Read the model definition and answer for the solid it produces. Units are mm, in the model's axes. Face numbers are marked on the shaded views. A direction names the side the tool comes from. Coordinates: 2 decimals unless noted, no trailing zeros. Write each loop counter-clockwise with the first axis right and the second up, starting at its lowest first coordinate (ties: lowest second). Pieces come first, ordered by that corner, then holes. Notation, with made-up numbers: (82.25, 72.5) -> (108.25, 72.5) arc R25 cw to (108.25, 96.5) -> close; hole circle Ø10 at (5, -0.75). An arc over 180 degrees is marked (long way). Use CSV: the item, a comma, the result in double quotes.
from build123d import *

# Parameters (mm, degrees)
F0_W     = 15
F0_H     = 18
F0_R     = 6
F0_W_2   = 10.2
F0_H_2   = 3.3
F1_DEPTH = 50
F2_D     = 12
F2_DEPTH = 45
F2_TIP   = 3.6051637142
F3_R     = 5
F4_R     = 5
F6_W     = 10.2
F6_H     = 3.3
F7_DEPTH = 40


with BuildPart() as f1:
    # F0 (on Top) → F1 (new body)
    with BuildSketch(Plane.XY):
        with Locations((0, 1.5)):
            Rectangle(F0_W, F0_H)
        Circle(F0_R, mode=Mode.SUBTRACT)
        with Locations((-0.15, 8.3)):
            Rectangle(F0_W_2, F0_H_2, mode=Mode.SUBTRACT)
        with Locations((-0.15, 8.3)):
            Rectangle(F0_W_2, F0_H_2)
        Circle(F0_R)
    extrude(amount=F1_DEPTH)

    # F2
    with Locations(Plane(origin=(0, 0, 0), x_dir=(1, 0, 0), z_dir=(0, 0, -1))):
        with Locations((0, 0)):
            Hole(F2_D / 2, depth=F2_DEPTH)
            with Locations((0, 0, -(F2_DEPTH + F2_TIP / 2))):  # 118° drill point
                Cone(0, F2_D / 2, F2_TIP, mode=Mode.SUBTRACT)

    # F3
    f3_edges = [f1.edges().sort_by_distance(p)[0] for p in [
        (7.5, -7.5, 25),
        (-7.5, -7.5, 25),
    ]]
    fillet(f3_edges, radius=F3_R)

    # F4
    f4_edges = [f1.edges().sort_by_distance(p)[0] for p in [
        (-7.5, 4, 50),
    ]]
    fillet(f4_edges, radius=F4_R)

    # F6 (on offset) → F7 (cut)
    with BuildSketch(Plane.XY.offset(50)):
        with Locations((0.15, 8.3)):
            Rectangle(F6_W, F6_H)
    extrude(amount=-F7_DEPTH, mode=Mode.SUBTRACT)


solid = f1.part
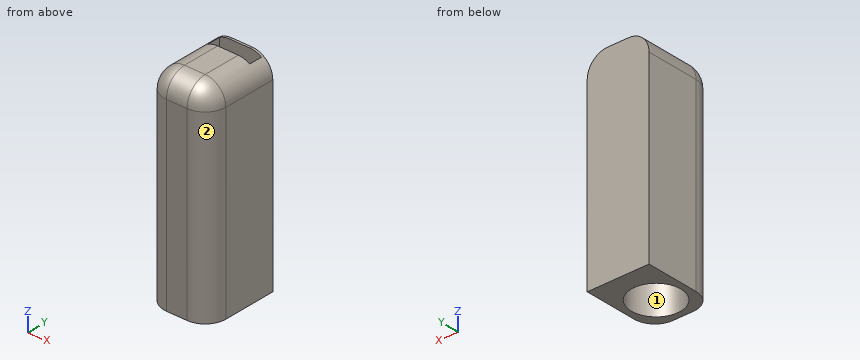
1. A tool of negligible diameter and unlimited length cuts with its end or side. For the marked faces 1 and 2, from which of +Z, -Z, +X, -X, +Y, -Y can it reach the whole face along a straight path? Write none if from no direction.
Solutions:
face 1,"-Z"
face 2,"+Z, -Z, +X, -Y"
2. Each of these flat-tipped pins is pushed along its axis until it touches: pin 1 Ø7 at (x, y) = (0, 0) entering from -Z; pin 2 Ø1.7 at (x, y) = (-0.5, 8.5) entering from +Z. Where does it stop, or does it pass through?
Solutions:
pin 1,"stops at z = 46.5"
pin 2,"stops at z = 10"
3. A cutting plane is placed at A-A (z = 19). Give the vertices of the cut face in (x, y).
Solutions:
outline,"(-7.5, -2.5) arc R5 ccw to (-2.5, -7.5) -> (2.5, -7.5) arc R5 ccw to (7.5, -2.5) -> (7.5, 10.5) -> (-7.5, 10.5) -> close; hole circle Ø12 at (0, 0); hole (-4.95, 6.65) -> (5.25, 6.65) -> (5.25, 9.95) -> (-4.95, 9.95) -> close"
4. Find the intervals of material crossed by line 1 along Y through (x, z) = (0, 22.5); line 2 along X through (y, z) = (9.5, 28); line 3 along Y through (x, z) = (-3.75, 43), in increasing order.
Solutions:
line 1,"y = -7.5 to -6, 6 to 6.65, 9.95 to 10.5"
line 2,"x = -7.5 to -4.95, 5.25 to 7.5"
line 3,"y = -7.34 to -4.68, 4.68 to 6.65, 9.95 to 10.5"
